from build123d import *

# Parameters (mm, degrees)
SKETCH1_W           = 20.5
SKETCH1_H           = 24
SKETCH1_R           = 1.3
BOSS_EXTRUDE1_DEPTH = 3.5
SKETCH2_W           = 2
SKETCH2_H           = 18.5
BOSS_EXTRUDE2_DEPTH = 24
SKETCH3_W           = 6.5
SKETCH3_H           = 10.5
BOSS_EXTRUDE3_DEPTH = 2
FILLET1_R           = 3.5
FILLET2_R           = 2
SKETCH4_R           = 2.25
CUT_EXTRUDE1_DEPTH  = 1.5
FILLET4_R           = 3
SKETCH13_W          = 24.5
SKETCH13_H          = 7.7
CUT_EXTRUDE6_DEPTH  = 25
BOSS_EXTRUDE6_START = -2
BOSS_EXTRUDE6_DEPTH = 2
BOSS_EXTRUDE7_DEPTH = 2


with BuildPart() as part:
    # Sketch1 → Boss-Extrude1 (new body)
    with BuildSketch(Plane.XY):
        with Locations((0, 1)):
            Rectangle(SKETCH1_W, SKETCH1_H)
        with Locations((-4.8, 5)):
            Circle(SKETCH1_R, mode=Mode.SUBTRACT)
        with Locations((4.8, 5)):
            Circle(SKETCH1_R, mode=Mode.SUBTRACT)
    extrude(amount=BOSS_EXTRUDE1_DEPTH)

    # Sketch2 → Boss-Extrude2 (add)
    with BuildSketch(Plane(origin=(0, -11, 0), x_dir=(-1, 0, 0), z_dir=(0, -1, 0))):
        with Locations((11.25, 5.75)):
            Rectangle(SKETCH2_W, SKETCH2_H)
        with Locations((-11.25, 5.75)):
            Rectangle(SKETCH2_W, SKETCH2_H)
    extrude(amount=-BOSS_EXTRUDE2_DEPTH)

    # Sketch3 → Boss-Extrude3 (add)
    with BuildSketch(Plane.XZ.offset(11)):
        with Locations((-7, -5.25)):
            Rectangle(SKETCH3_W, SKETCH3_H)
        with Locations((7, -5.25)):
            Rectangle(SKETCH3_W, SKETCH3_H)
    extrude(amount=-BOSS_EXTRUDE3_DEPTH)

    # Fillet1
    fillet1_edges = [part.edges().sort_by_distance(p)[0] for p in [
        (-3.75, -10, 0),
        (3.75, -10, 0),
    ]]
    fillet(fillet1_edges, radius=FILLET1_R)

    # Fillet2
    fillet2_edges = [part.edges().sort_by_distance(p)[0] for p in [
        (-12.25, 1, 3.5),
        (12.25, 1, 3.5),
    ]]
    fillet(fillet2_edges, radius=FILLET2_R)

    # Sketch4 → Cut-Extrude1 (cut)
    with BuildSketch(Plane.XY.offset(3.5)):
        with Locations((-4.8, 5)):
            Circle(SKETCH4_R)
        with Locations((4.8, 5)):
            Circle(SKETCH4_R)
    extrude(amount=-CUT_EXTRUDE1_DEPTH, mode=Mode.SUBTRACT)

    # Fillet4
    fillet4_edges = [part.edges().sort_by_distance(p)[0] for p in [
        (-11.25, 13, -15),
        (11.25, 13, -15),
        (11.25, -11, -15),
    ]]
    fillet(fillet4_edges, radius=FILLET4_R)

    # Sketch13 → Cut-Extrude6 (cut, through all)
    with BuildSketch(Plane(origin=(0, 13, 0), x_dir=(1, 0, 0), z_dir=(0, 1, 0))):
        with Locations((0, 11.15)):
            Rectangle(SKETCH13_W, SKETCH13_H)
    extrude(amount=-CUT_EXTRUDE6_DEPTH, mode=Mode.SUBTRACT)

    # Sketch14 → Boss-Extrude6 (add)
    with BuildSketch(Plane.XZ.offset(11).offset(BOSS_EXTRUDE6_START)):
        with BuildLine():
            Line((-0.25, 0), (0.25, 0))
            ThreePointArc((0.25, 0), (2.668052064, -0.969580229), (3.746392428, -3.341129019))
            Line((3.746392428, -3.341129019), (1.948302942, -3.341129019))
            ThreePointArc((1.948302942, -3.341129019), (0, -1.545230361), (-1.948302942, -3.341129019))
            Line((-1.948302942, -3.341129019), (-3.746392428, -3.341129019))
            ThreePointArc((-3.746392428, -3.341129019), (-2.668052064, -0.969580229), (-0.25, 0))
        make_face()
    extrude(amount=BOSS_EXTRUDE6_DEPTH)

    # Sketch15 → Boss-Extrude7 (add)
    with BuildSketch(Plane(origin=(0, -11, 0), x_dir=(-1, 0, 0), z_dir=(0, -1, 0))):
        with BuildLine():
            Line((1.948302942, 3.341129019), (3.746392428, 3.341129019))
            ThreePointArc((3.746392428, 3.341129019), (0, -0.246607561), (-3.746392428, 3.341129019))
            Line((-3.746392428, 3.341129019), (-1.948302942, 3.341129019))
            ThreePointArc((-1.948302942, 3.341129019), (0, 1.545230361), (1.948302942, 3.341129019))
        make_face()
    extrude(amount=BOSS_EXTRUDE7_DEPTH)


solid = part.part
CAD build for the part. Positions are in the model's coordinates, mm. A direction names the side the tool comes from. Coordinates: 2 decimals unless noted, no trailing zeros. Order: outer loops, then holes, each group sorted by start corner. A loop starts at its lowest first (then second) coordinate and runs counter-clockwise, first axis right, second up.
Item 1: Band-saw the part on C-C on x = 0. List the corners of the cut face in (y, z).
Check sheet entries:
outline: (-13, -1.55) - (-9, -1.55) - (-9, 0) - (13, 0) - (13, 3.5) - (-11, 3.5) - (-11, 0.25) - (-13, 0.25) - close
Item 2: Drill centre lines: L1, parallel to X at y = 5, z = 0.8; L2, parallel to X at y = 10.5, z = -1.5; L3, parallel to Y at x = 4.8, z = 2.8. Where is each one in solid material? Low to high.
Check sheet entries:
L1: x = -12.25 to -6.1, -3.5 to 3.5, 6.1 to 12.25
L2: x = -12.25 to -10.25, 10.25 to 12.25
L3: y = -11 to 2.75, 7.25 to 13
Item 3: Band-saw the part on D-D on y = -3.25. List the corners of the cut face in (x, z), plus the area to 3 significant figures.
Check sheet entries:
outline: (-12.25, -7.3) - (-10.25, -7.3) - (-10.25, 0) - (10.25, 0) - (10.25, -7.3) - (12.25, -7.3) - (12.25, 1.5) arc R2 ccw to (10.25, 3.5) - (-10.25, 3.5) arc R2 ccw to (-12.25, 1.5) - close
area: 113 mm2
Item 4: Band-saw the part on A-A on x = -4.8. List the corners of the cut face in (y, z).
Check sheet entries:
outline: (-11, -7.3) - (-9, -7.3) - (-9, 0) - (3.7, 0) - (3.7, 2) - (2.75, 2) - (2.75, 3.5) - (-11, 3.5) - close; (6.3, 0) - (13, 0) - (13, 3.5) - (7.25, 3.5) - (7.25, 2) - (6.3, 2) - close
Item 5: Pin check, flat tips, straight feed: pin 1 Ø2 at (x, z) = (9, -4) entering from +Y; pin 2 Ø3.5 at (x, y) = (-4.8, 5) entering from +Z; pin 3 Ø4 at (x, z) = (4, -6) entering from -Y. Stop position of each tip, or through.
Check sheet entries:
pin 1: stops at y = -9
pin 2: stops at z = 2
pin 3: stops at y = -11
Item 6: 3-axis set-ups, long thin cutter, end or side, ignore diameter. For faces 1 (the face through (3.75, -10, -5)), 2 (the face through (12.25, 1, -3)), 3 (the face through (10.25, 2, -4)), 4 (the face through (10.5, -1.6, -7.3)), 5 (the face through (-4.8, 3.5, 2)): which of +Z, -Z, +X, -X, +Y, -Y reach the whole face in a straight line?
Check sheet entries:
face 1: -Z, +Y, -Y
face 2: +Z, -Z, +X, +Y, -Y
face 3: -Z, +Y
face 4: -Z, +X, -X, +Y, -Y
face 5: +Z
Item 7: Band-saw the part on B-B on z = -6. List the corners of the cut face in (x, y).
Check sheet entries:
outline: (-12.25, -11) - (-3.75, -11) - (-3.75, -9) - (-10.25, -9) - (-10.25, 13) - (-12.25, 13) - close; (3.75, -11) - (12.25, -11) - (12.25, 13) - (10.25, 13) - (10.25, -9) - (3.75, -9) - close
Item 8: Two-plate mould, pull along Y, no slides. Class faces 6 (the face through (0.2, 13, 0.4)), 7 (the face through (0, -13, -1)), 8 (the face through (11.65, 1.17, 2.93)), 9 (the face through (5.4, 3.847, 0.986)): +Y half, -Y half, draft (parallel to the pull), parting line (faces both ways), or undercut.
Check sheet entries:
face 6: +Y half
face 7: -Y half
face 8: draft
face 9: undercut
